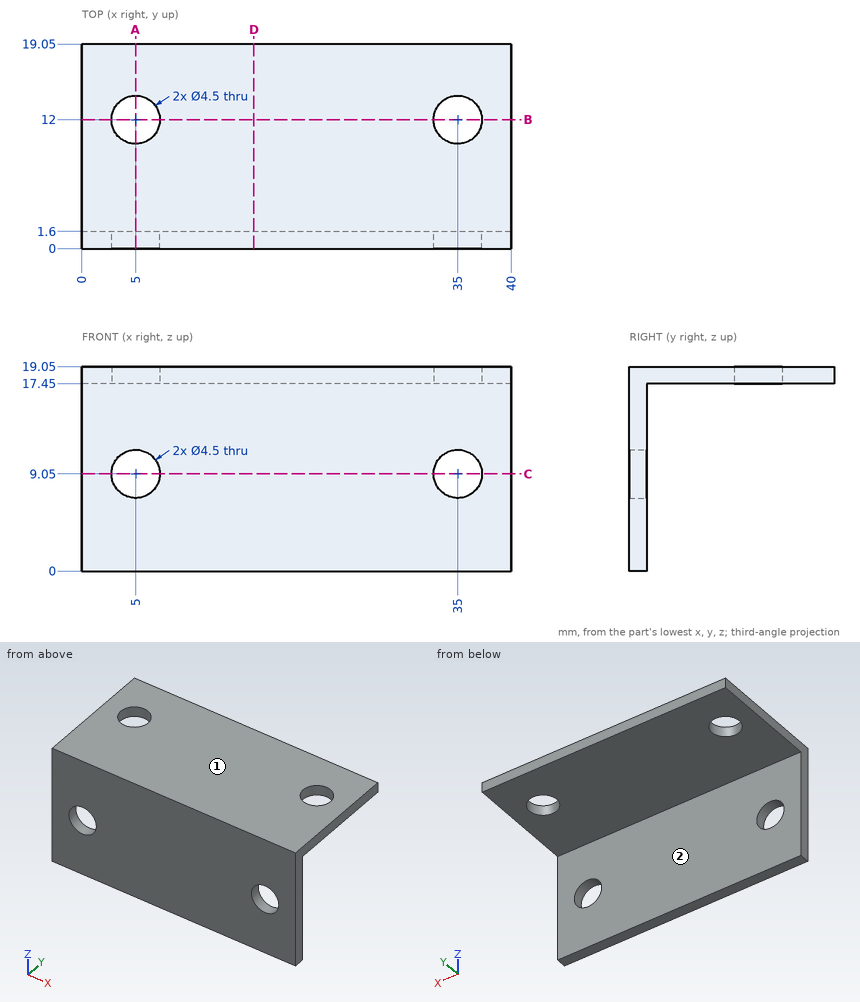
Drawing for the job (mm, zero at the part's lowest x, y, z). A direction names the side the tool comes from. Round coordinates to 2 decimals unless told otherwise and drop trailing zeros. Order: outer loops, then holes, each group sorted by start corner. A loop starts at its lowest first (then second) coordinate and runs counter-clockwise, first axis right, second up.
Item 1: Saw through at C-C on z = 9.05. Write the cut outline in (x, y), then the cut area to 3 significant figures.
Item 2: Tool access for the marked faces 1 and 2: list every direction of +Z, -Z, +X, -X, +Y, -Y with a clear straight run to the whole face (end or side of a thin tool).
Item 3: Pin check, flat tips, straight feed: pin 1 (10 mm diameter, centred on y = 10.5, z = 11, fed in from +X); pin 2 (8.5 mm diameter, centred on x = 16, z = 12.5, fed in from +Y); pin 3 (5 mm diameter, centred on x = 5, y = 12, fed in from +Z); pin 4 (3 mm diameter, centred on x = 34, y = 11.5, fed in from -Z). Stop position of each tip, or through.
Item 4: Probe line 1 along X through (y, z) = (1, 9.05); line 2 along Z through (x, y) = (35, 0.55); line 3 along Y through (x, z) = (15, 6). List the from-to ranges inside material, lowest first.
Item 5: Saw through at D-D on x = 16. Write the cut outline in (y, z), then the cut area to 3 significant figures.
Item 6: Saw through at A-A on x = 5. Write the cut outline in (y, z), then the cut area to 3 significant figures.
Item 7: Saw through at B-B on y = 12. Write the cut outline in (x, z), then the cut area to 3 significant figures.
Reported:
1. outline: (0, 0) - (2.75, 0) - (2.75, 1.6) - (0, 1.6) - close; (7.25, 0) - (32.75, 0) - (32.75, 1.6) - (7.25, 1.6) - close; (37.25, 0) - (40, 0) - (40, 1.6) - (37.25, 1.6) - close
1. area: 49.6 mm2
2. face 1: +Z, +X, -X, +Y, -Y
2. face 2: -Z, +X, -X, +Y
3. pin 1: passes through
3. pin 2: stops at y = 1.6
3. pin 3: stops at z = 19.05
3. pin 4: stops at z = 17.45
4. line 1: x = 0 to 2.75, 7.25 to 32.75, 37.25 to 40
4. line 2: z = 0 to 6.8, 11.3 to 19.05
4. line 3: y = 0 to 1.6
5. outline: (0, 0) - (1.6, 0) - (1.6, 17.45) - (19.05, 17.45) - (19.05, 19.05) - (0, 19.05) - close
5. area: 58.4 mm2
6. outline: (0, 0) - (1.6, 0) - (1.6, 6.8) - (0, 6.8) - close; (0, 11.3) - (1.6, 11.3) - (1.6, 17.45) - (9.75, 17.45) - (9.75, 19.05) - (0, 19.05) - close; (14.25, 17.45) - (19.05, 17.45) - (19.05, 19.05) - (14.25, 19.05) - close
6. area: 44.0 mm2
7. outline: (0, 17.45) - (2.75, 17.45) - (2.75, 19.05) - (0, 19.05) - close; (7.25, 17.45) - (32.75, 17.45) - (32.75, 19.05) - (7.25, 19.05) - close; (37.25, 17.45) - (40, 17.45) - (40, 19.05) - (37.25, 19.05) - close
7. area: 49.6 mm2
